Here's how the part is built. I have some questions about the finished solid (model axes, mm). A direction names the side the tool comes from. Round coordinates to 2 decimals unless told otherwise and drop trailing zeros. Loops run counter-clockwise (first coordinate to the right, second up) from the corner with the lowest first, then second, coordinate; pieces in that order, holes last. Notation, with made-up numbers: M 38.5,-26 L 52.5,-26 A24 cw 52.5,5 Z; hole C 88.5,32.25 d11. An arc over 180 degrees is marked long. Answer as a JSON object with one key per item and string values.
from build123d import *

# Parameters (mm, degrees)
SKETCH1_W               = 58
SKETCH1_H               = 38.77382393
SKETCH1_W_2             = 42
SKETCH1_H_2             = 21.5
BOSS_EXTRUDE2_DEPTH     = 38.65
CUT_EXTRUDE3_DEPTH      = 71.201780604
BOSS_EXTRUDE3_REACH     = 72.202
CUT_EXTRUDE5_DEPTH      = 71.201780604
SKETCH10_W              = 5.5
SKETCH10_H              = 7
CUT_EXTRUDE6_DEPTH      = 17
FILLET1_R               = 1
CUT_EXTRUDE7_DEPTH      = 50.043755974
CUT_EXTRUDE7_DEPTH_BACK = 20
SKETCH11_R              = 15.5
SKETCH12_R              = 3
CUT_EXTRUDE8_DEPTH      = 20
SKETCH13_R              = 4
CUT_EXTRUDE9_DEPTH      = 20
SKETCH15_R              = 1
CUT_EXTRUDE10_DEPTH     = 10
CUT_EXTRUDE11_DEPTH     = 55.764153522


with BuildPart() as part:
    # Sketch1 → Boss-Extrude2 (new body)
    with BuildSketch(Plane(origin=(0, -30, 0), x_dir=(1, 0, 0), z_dir=(0, 1, 0))):
        with Locations((0, -6.386911965)):
            Rectangle(SKETCH1_W, SKETCH1_H)
        with Locations((0, -0.25)):
            Rectangle(SKETCH1_W_2, SKETCH1_H_2, mode=Mode.SUBTRACT)
    extrude(amount=BOSS_EXTRUDE2_DEPTH)

    # Sketch6 → Cut-Extrude3 (cut, through all)
    with BuildSketch(Plane(origin=(29, 0, 0), x_dir=(0, 0, -1), z_dir=(1, 0, 0))):
        Polygon((-11, -30), (-4, -8), (9, -8), (13, -5), (13, -30), align=None)
    extrude(amount=-CUT_EXTRUDE3_DEPTH, mode=Mode.SUBTRACT)

    # Boss-Extrude3: up to this face of the body (flat: up to its plane)
    boss_extrude3_end = Plane(part.part.faces().sort_by_distance((29, -6.820520007, 10.403923083))[0])
    # Sketch9 → Boss-Extrude3 (add, up to the picked face)
    with BuildSketch(Plane.ZY.offset(29), mode=Mode.PRIVATE) as boss_extrude3_sk1:
        Polygon((10.77382393, 8.65), (18.77382393, 20.15), (25.77382393, 20.15), (25.77382393, 8.65), align=None)
    boss_extrude3_tool1 = split(extrude(boss_extrude3_sk1.sketch, amount=-BOSS_EXTRUDE3_REACH, mode=Mode.PRIVATE), bisect_by=boss_extrude3_end, keep=Keep.BOTH, mode=Mode.PRIVATE)
    add(boss_extrude3_tool1.solids().sort_by(Axis((-29, 13.70303, 20.0314), (1, 0, 0)))[0])

    # Sketch8 → Cut-Extrude5 (cut, through all)
    with BuildSketch(Plane.ZY.offset(29)):
        Polygon((25.77382393, 9.78375673), (13.27382393, 2.566878365), (13.27382393, -11.866878365), (25.77382393, -19.08375673), (38.27382393, -11.866878365), (38.27382393, 2.566878365), align=None)
    extrude(amount=-CUT_EXTRUDE5_DEPTH, mode=Mode.SUBTRACT)

    # Sketch10 → Cut-Extrude6 (cut)
    with BuildSketch(Plane(origin=(0, 20.15, 0), x_dir=(1, 0, 0), z_dir=(0, 1, 0))):
        with BuildLine():
            Line((-4.2, -12.77382393), (-4.2, -15.123119728))
            ThreePointArc((-4.2, -15.123119728), (-1.45, -14.77382393), (1.3, -15.123119728))
            Line((1.3, -15.123119728), (1.3, -12.77382393))
            Line((1.3, -12.77382393), (-4.2, -12.77382393))
        make_face()
        with BuildLine():
            Line((1.3, -18.77382393), (1.3, -25.77382393))
            Line((1.3, -25.77382393), (9.55, -25.77382393))
            ThreePointArc((9.55, -25.77382393), (8.90224843, -22.054825081), (7.035281374, -18.77382393))
            Line((7.035281374, -18.77382393), (1.3, -18.77382393))
        make_face()
        with BuildLine():
            Line((1.3, -15.123119728), (1.3, -18.77382393))
            Line((1.3, -18.77382393), (7.035281374, -18.77382393))
            ThreePointArc((7.035281374, -18.77382393), (4.456758602, -16.4942656), (1.3, -15.123119728))
        make_face()
        with BuildLine():
            Line((-4.2, -15.123119728), (-4.2, -18.77382393))
            Line((-4.2, -18.77382393), (1.3, -18.77382393))
            Line((1.3, -18.77382393), (1.3, -15.123119728))
            ThreePointArc((1.3, -15.123119728), (-1.45, -14.77382393), (-4.2, -15.123119728))
        make_face()
        with BuildLine():
            Line((-12.45, -25.77382393), (-4.2, -25.77382393))
            Line((-4.2, -25.77382393), (-4.2, -18.77382393))
            Line((-4.2, -18.77382393), (-9.935281374, -18.77382393))
            ThreePointArc((-9.935281374, -18.77382393), (-11.80224843, -22.054825081), (-12.45, -25.77382393))
        make_face()
        with Locations((-1.45, -22.27382393)):
            Rectangle(SKETCH10_W, SKETCH10_H)
        with BuildLine():
            Line((-9.935281374, -18.77382393), (-4.2, -18.77382393))
            Line((-4.2, -18.77382393), (-4.2, -15.123119728))
            ThreePointArc((-4.2, -15.123119728), (-7.356758602, -16.4942656), (-9.935281374, -18.77382393))
        make_face()
    extrude(amount=-CUT_EXTRUDE6_DEPTH, mode=Mode.SUBTRACT)

    # Fillet1
    fillet1_edges = [part.edges().sort_by_distance(p)[0] for p in [
        (1.3, 7.3375, 12.77382393),
        (-4.2, 7.3375, 12.77382393),
    ]]
    fillet(fillet1_edges, radius=FILLET1_R)

    # Sketch11 → Cut-Extrude7 (cut, two sides: drawn at the far end of the back side and taken through both)
    with BuildSketch(Plane(origin=(0, 0, 0), x_dir=(0, 0, -1), z_dir=(1, 0, 0)).offset(-CUT_EXTRUDE7_DEPTH_BACK)):
        with Locations((-25.77382393, -4.65)):
            Circle(SKETCH11_R)
    extrude(amount=CUT_EXTRUDE7_DEPTH + CUT_EXTRUDE7_DEPTH_BACK, mode=Mode.SUBTRACT)

    # Sketch12 → Cut-Extrude8 (cut)
    with BuildSketch(Plane.XY.offset(25.77382393)):
        with Locations((-22, 14.966878365)):
            Circle(SKETCH12_R)
        with Locations((22, 14.966878365)):
            Circle(SKETCH12_R)
        with Locations(Location((22, -24.816878365, 0), (0, 0, 250.528779366))):
            Circle(SKETCH12_R)
        with Locations(Location((-22, -24.816878365, 0), (0, 0, 70.528779366))):
            Circle(SKETCH12_R)
    extrude(amount=-CUT_EXTRUDE8_DEPTH, mode=Mode.SUBTRACT)

    # Sketch13 → Cut-Extrude9 (cut)
    with BuildSketch(Plane.XY):
        with Locations(Location((22, 14.966878365, 0), (0, 0, 270))):
            Circle(SKETCH13_R)
        with Locations(Location((-22, 14.966878365, 0), (0, 0, 270))):
            Circle(SKETCH13_R)
        with Locations(Location((22, -24.816878365, 0), (0, 0, 255.522487814))):
            Circle(SKETCH13_R)
        with Locations(Location((-22, -24.816878365, 0), (0, 0, 75.522487814))):
            Circle(SKETCH13_R)
    extrude(amount=CUT_EXTRUDE9_DEPTH, mode=Mode.SUBTRACT)

    # Sketch15 → Cut-Extrude10 (cut)
    with BuildSketch(Plane(origin=(0, 8.65, 0), x_dir=(1, 0, 0), z_dir=(0, 1, 0))):
        with Locations(Location((-24.3, 5, 0), (0, 0, 270))):
            Circle(SKETCH15_R)
        with Locations(Location((-24.3, -5, 0), (0, 0, 90))):
            Circle(SKETCH15_R)
        with Locations(Location((24.2, 5, 0), (0, 0, 270))):
            Circle(SKETCH15_R)
        with Locations(Location((24.2, -5, 0), (0, 0, 90))):
            Circle(SKETCH15_R)
    extrude(amount=-CUT_EXTRUDE10_DEPTH, mode=Mode.SUBTRACT)

    # Sketch17 → Cut-Extrude11 (cut, through all)
    with BuildSketch(Plane(origin=(0, 8.65, 0), x_dir=(1, 0, 0), z_dir=(0, 1, 0))):
        Polygon((-21, -3.5), (-21, 3.5), (-23.1, 2.75), (-23.1, -2.75), align=None)
    extrude(amount=-CUT_EXTRUDE11_DEPTH, mode=Mode.SUBTRACT)


solid = part.part
Item 1: I'm going to push flat-ended pins straight in: pin 1 Ø4 at (x, y) = (21, -23) entering from -Z; pin 2 Ø9 at (x, z) = (-24.5, -2) entering from -Y; pin 3 Ø2 at (x, z) = (24.5, -4.5) entering from +Y. Where does each tip first touch, or does it pass through?
Resolved:
{"pin 1": "z = 11", "pin 2": "y = -8", "pin 3": "y = 8.65"}
Item 2: I want a section at C-C, the plane x = -22. State how many separate pieces and enclosed holes the cut face has, then the cut area to 3 significant figures.
Resolved:
{"separate pieces": "4", "enclosed holes": "0", "area": "600 mm²"}
Item 3: Please list where these lines run through material, in increasing order: probe 1 along X at (y, z) = (3.25, -5); probe 2 along X at (y, z) = (-6, -8); probe 3 along Y at (x, z) = (-22, 22.2). Write a range as from..to.
Resolved:
{"probe 1": "-29..-25.3, -23.3..-21, 21..23.2, 25.2..29", "probe 2": "-29..-21, 21..29", "probe 3": "-30..-27.82, -21.82..-17.02, 7.72..11.97, 17.97..20.15"}
Item 4: I want a section at B-B, the plane z = 17. Please give me the cut outline in (x, y), then the cut area to 3 significant figures.
Resolved:
{"outline": "M -29,-30 L 29,-30 L 29,-17.43 L -20,-17.43 L -20,-14.02 L -29,-14.02 Z; M -29,4.72 L -20,4.72 L -20,8.13 L -8.08,8.13 L -8.08,17.6 L -18.99,17.6 A4 cw long -25.01,17.6 L -29,17.6 Z; M 5.18,8.13 L 29,8.13 L 29,17.6 L 25.01,17.6 A4 cw long 18.99,17.6 L 5.18,17.6 Z; hole C -22,-24.82 d8; hole C 22,-24.82 d8", "area": "1,020 mm²"}
Item 5: On a 3-axis mill with a long thin cutter (end or side, diameter ignored), from which of +Z, -Z, +X, -X, +Y, -Y can I reach the whole of each face in a straight line? I mean faces 3 (the face through (0, 8.65, -11)), 4 (the face through (-23.1, 0, 0)), 5 (the face through (-25.19, 3.72, -4.54)), 6 (the face through (23.2, 11.15, 16.99)). Say none if no direction works.
Resolved:
{"face 3": "-Z, +X, -X, +Y", "face 4": "+Y, -Y", "face 5": "+Y", "face 6": "-Z"}
Item 6: I want a section at D-D, the plane x = 22. Please give me the cut outline in (y, z), then the cut area to 3 significant figures.
Resolved:
{"outline": "M -30,11 L -28.82,10.62 L -28.82,20 L -27.82,20 L -27.82,25.77 L -30,25.77 Z; M -21.82,20 L -20.82,20 L -20.82,8.08 L -8,4 L -8,-9 L -5,-13 L 8.65,-13 L 8.65,10.77 L 10.97,12.39 L 10.97,20 L 11.97,20 L 11.97,25.77 L 10.85,25.77 A15.5 cw -20.15,25.77 L -21.82,25.77 Z; M 17.97,20 L 18.97,20 L 18.97,17.95 L 20.15,18.77 L 20.15,25.77 L 17.97,25.77 Z", "area": "598 mm²"}
Item 7: I want a section at A-A, the plane z = -5. Please give me the cut outline in (x, y), then the cut area to 3 significant figures.
Resolved:
{"outline": "M -29,-8 L -21,-8 L -21,8.65 L -23.3,8.65 L -23.3,-1.35 L -25.3,-1.35 L -25.3,8.65 L -29,8.65 Z; M 21,-8 L 29,-8 L 29,8.65 L 25.2,8.65 L 25.2,-1.35 L 23.2,-1.35 L 23.2,8.65 L 21,8.65 Z", "area": "226 mm²"}
Item 8: If we mould it in two halves opening along X, with no side actions, what happens to faces 1 (the face through (19, 17, 25.774)), 2 (the face through (-22.04, 0.44, -3.13))? For each: pulls with the +X half, pulls with the -X half, needs draft (parallel to the pull), parting line crosses it, or undercut.
Resolved:
{"face 1": "needs draft", "face 2": "undercut"}
